Could you check a few things on this model? Use its own coordinates, in mm. A direction names the side the tool comes from. Round coordinates to 2 decimals unless told otherwise and drop trailing zeros. Loops run counter-clockwise (first coordinate to the right, second up) from the corner with the lowest first, then second, coordinate; pieces in that order, holes last. Notation, with made-up numbers: (23.25, -23) -> (78.25, -23) arc R10 ccw to (78.25, -17) -> close; hole circle Ø11 at (11.25, -4). An arc over 180 degrees is marked (long way). Write each question's results on one line, items separated by ' | '.
Autodesk Inventor part; units mm, degrees
ref_plane "YZ Plane" through (0, 0, 0) normal (1, 0, 0) x (0, 1, 0)
ref_plane "XZ Plane" through (0, 0, 0) normal (0, 1, 0) x (-1, 0, 0)
ref_plane "XY Plane" through (0, 0, 0) normal (0, 0, 1) x (1, 0, 0)
sketch "Sketch1" plane through (0, 0, 0) normal (0, 1, 0) x (-1, 0, 0)
  line L0 (0, 0) -> (-10, 0) construction
  line L1 (-10, 0) -> (-10, -10)
  line L2 (-10, -10) -> (0, -10)
  line L3 (0, -10) -> (0, 0) construction
  line L4 (-10, 0) -> (-10, 10)
  line L5 (-10, 10) -> (0, 10)
  line L6 (10, 0) -> (10, -10)
  line L7 (10, -10) -> (0, -10)
  line L8 (10, 10) -> (0, 10)
  line L9 (10, 0) -> (10, 10)
  dimension "d0" = 10
extrude "Extrusion1" add sketch "Sketch1" along normal mid plane 10
sketch "Sketch2" plane through (-10, 5, 10) normal (0, 0, 1) x (1, 0, 0)
  circle A0 centre (10, -5) radius 5
  dimension "d4" = 10
extrude "Extrusion2" add sketch "Sketch2" along normal blind 23.5
mirror "Mirror1" about plane through (0, 0, 0) normal (0, 0, 1) of "Extrusion2"
sketch "Sketch3" plane through (10, -5, -10) normal (1, 0, 0) x (0, 0, -1)
  circle A0 centre (-10, 5) radius 5
  dimension "d8" = 10
extrude "Extrusion3" add sketch "Sketch3" along normal blind 23.5
mirror "Mirror2" about plane through (0, 0, 0) normal (1, 0, 0) of "Extrusion3"
move or copy body "Move Body1" bodies to move or copy 1 copy no rotation origin (0, 0, 0) rotation axis (1, 0, 0) rotation angle 90
move or copy body "Move Body2" bodies to move or copy 1 copy no rotation origin (0, 0, 0) rotation axis (0, 0, 1) rotation angle 90
properties part number "AnkRoll_v2"
1) I want a section at A-A, the plane z = 4. Write out the boundary of the cut face in (x, y), plus the area to 3 significant figures.
Model answer:
outline: (-33.5, -3) -> (-10, -3) -> (-10, -10) -> (-3, -10) -> (-3, -33.5) -> (3, -33.5) -> (3, -10) -> (10, -10) -> (10, -3) -> (33.5, -3) -> (33.5, 3) -> (10, 3) -> (10, 10) -> (3, 10) -> (3, 33.5) -> (-3, 33.5) -> (-3, 10) -> (-10, 10) -> (-10, 3) -> (-33.5, 3) -> close | area: 964 mm2
2) I want a section at D-D, the plane z = 0. Write out the boundary of the cut face in (x, y), plus the area to 3 significant figures.
Model answer:
outline: (-33.5, -5) -> (-10, -5) -> (-10, -10) -> (-5, -10) -> (-5, -33.5) -> (5, -33.5) -> (5, -10) -> (10, -10) -> (10, -5) -> (33.5, -5) -> (33.5, 5) -> (10, 5) -> (10, 10) -> (5, 10) -> (5, 33.5) -> (-5, 33.5) -> (-5, 10) -> (-10, 10) -> (-10, 5) -> (-33.5, 5) -> close | area: 1,340 mm2
3) For faces 1 (the cylindrical face through (1.08, -21.59, -4.88)), 2 (the cylindrical face through (-21.59, -1.08, -4.88)), 3 (the cylindrical face through (1.08, 21.59, 4.88)), 4 (the flat face through (7, -10, 0)), which set-ups out of +Z, -Z, +X, -X, +Y, -Y let a thin tool reach every point of the face, with its end or its side?
Model answer:
face 1: -Y | face 2: -X | face 3: +Y | face 4: +X, -Y
4) I want a section at B-B, the plane y = 19.5. Write out the boundary of the cut face in (x, z), plus the area to 3 significant figures.
Model answer:
outline: circle Ø10 at (0, 0) | area: 78.5 mm2
5) I want a section at C-C, the plane x = 7. Write out the boundary of the cut face in (y, z).
Model answer:
outline: (-10, -5) -> (10, -5) -> (10, 5) -> (-10, 5) -> close
6) I need wall thicknesses on line 1 (X direction, y = 9, z = -3.5); line 2 (Y direction, x = 25, z = -3.5). Which ranges of each line are inside material? Lowest first, please.
Model answer:
line 1: x = -10 to 10 | line 2: y = -3.57 to 3.57
7) I'm going to push flat-ended pins straight in: pin 1 (1 mm diameter, centred on x = -21.5, z = -3.5, fed in from +Y); pin 2 (4 mm diameter, centred on y = -10, z = 0.5, fed in from +X); pin 3 (6 mm diameter, centred on x = 25.5, z = -1, fed in from +Y). Where does each tip first touch, or does it pass through?
Model answer:
pin 1: stops at y = 4 | pin 2: stops at x = 10 | pin 3: stops at y = 5
